Build history of the part. All positions in model axes, mm. A direction names the side the tool comes from. Round coordinates to 2 decimals unless told otherwise and drop trailing zeros. Write each loop counter-clockwise with the first axis right and the second up, starting at its lowest first coordinate (ties: lowest second). Pieces come first, ordered by that corner, then holes.
from build123d import *

# Parameters (mm, degrees)
SKETCH1_W           = 98
SKETCH1_H           = 60
BOSS_EXTRUDE1_DEPTH = 1.5
SKETCH2_W           = 87.5
SKETCH2_H           = 42
BOSS_EXTRUDE2_DEPTH = 9
SKETCH3_W           = 76.5
SKETCH3_H           = 25.4
CUT_EXTRUDE1_DEPTH  = 0.5
SKETCH4_R           = 1.25
CUT_EXTRUDE2_DEPTH  = 116.260574352
SKETCH5_R           = 0.5
CUT_EXTRUDE3_DEPTH  = 10
BOSS_EXTRUDE3_START = 0.1
SKETCH6_R           = 0.75
SKETCH6_R_2         = 0.5
SKETCH6_W           = 1.5
SKETCH6_H           = 1.5
BOSS_EXTRUDE3_DEPTH = 0.1
SKETCH7_R           = 0.75
SKETCH7_R_2         = 0.5
SKETCH7_W           = 1.5
SKETCH7_H           = 1.5
BOSS_EXTRUDE4_DEPTH = 1.7
BOSS_EXTRUDE5_DEPTH = 2.59


with BuildPart() as part:
    # Sketch1 → Boss-Extrude1 (new body)
    with BuildSketch(Plane(origin=(0, 0, 0), x_dir=(1, 0, 0), z_dir=(0, 1, 0))):
        with Locations((49, 30)):
            Rectangle(SKETCH1_W, SKETCH1_H)
    extrude(amount=BOSS_EXTRUDE1_DEPTH)

    # Sketch2 → Boss-Extrude2 (add)
    with BuildSketch(Plane(origin=(0, 1.5, 0), x_dir=(1, 0, 0), z_dir=(0, 1, 0))):
        with Locations((49, 30)):
            Rectangle(SKETCH2_W, SKETCH2_H)
    extrude(amount=BOSS_EXTRUDE2_DEPTH)

    # Sketch3 → Cut-Extrude1 (cut)
    with BuildSketch(Plane(origin=(0, 10.5, 0), x_dir=(1, 0, 0), z_dir=(0, 1, 0))):
        with Locations((49, 30)):
            Rectangle(SKETCH3_W, SKETCH3_H)
    extrude(amount=-CUT_EXTRUDE1_DEPTH, mode=Mode.SUBTRACT)

    # Sketch4 → Cut-Extrude2 (cut, through all)
    with BuildSketch(Plane(origin=(0, 1.5, 0), x_dir=(1, 0, 0), z_dir=(0, 1, 0))):
        with Locations(Location((2.5, 57.5, 0), (0, 0, 270))):
            Circle(SKETCH4_R)
        with Locations(Location((95.5, 57.5, 0), (0, 0, 270))):
            Circle(SKETCH4_R)
        with Locations(Location((95.5, 2.5, 0), (0, 0, 270))):
            Circle(SKETCH4_R)
        with Locations(Location((2.5, 2.5, 0), (0, 0, 270))):
            Circle(SKETCH4_R)
    extrude(amount=-CUT_EXTRUDE2_DEPTH, mode=Mode.SUBTRACT)

    # Sketch5 → Cut-Extrude3 (cut)
    with BuildSketch(Plane(origin=(0, 1.5, 0), x_dir=(1, 0, 0), z_dir=(0, 1, 0))):
        with Locations(Location((10, 57.5, 0), (0, 0, 270))):
            Circle(SKETCH5_R)
        with Locations(Location((12.54, 57.5, 0), (0, 0, 270))):
            Circle(SKETCH5_R)
        with Locations(Location((15.08, 57.5, 0), (0, 0, 270))):
            Circle(SKETCH5_R)
        with Locations(Location((20.16, 57.5, 0), (0, 0, 270))):
            Circle(SKETCH5_R)
        with Locations(Location((22.7, 57.5, 0), (0, 0, 270))):
            Circle(SKETCH5_R)
        with Locations(Location((25.24, 57.5, 0), (0, 0, 270))):
            Circle(SKETCH5_R)
        with Locations(Location((27.78, 57.5, 0), (0, 0, 270))):
            Circle(SKETCH5_R)
        with Locations(Location((30.32, 57.5, 0), (0, 0, 270))):
            Circle(SKETCH5_R)
        with Locations(Location((32.86, 57.5, 0), (0, 0, 270))):
            Circle(SKETCH5_R)
    extrude(amount=-CUT_EXTRUDE3_DEPTH, mode=Mode.SUBTRACT)

    # Sketch6 → Boss-Extrude3 (add)
    # profile 1 of 9: a face of its own
    with BuildSketch(Plane(origin=(0, 1.5, 0), x_dir=(1, 0, 0), z_dir=(0, 1, 0)).offset(BOSS_EXTRUDE3_START)):
        with Locations(Location((12.54, 57.5, 0), (0, 0, 90))):
            Circle(SKETCH6_R)
        with Locations(Location((12.54, 57.5, 0), (0, 0, 270))):
            Circle(SKETCH6_R_2, mode=Mode.SUBTRACT)
    # profile 2 of 9: a face of its own
    with BuildSketch(Plane(origin=(0, 1.5, 0), x_dir=(1, 0, 0), z_dir=(0, 1, 0)).offset(BOSS_EXTRUDE3_START)):
        with Locations(Location((15.08, 57.5, 0), (0, 0, 90))):
            Circle(SKETCH6_R)
        with Locations(Location((15.08, 57.5, 0), (0, 0, 270))):
            Circle(SKETCH6_R_2, mode=Mode.SUBTRACT)
    # profile 3 of 9: a face of its own
    with BuildSketch(Plane(origin=(0, 1.5, 0), x_dir=(1, 0, 0), z_dir=(0, 1, 0)).offset(BOSS_EXTRUDE3_START)):
        with Locations(Location((22.7, 57.5, 0), (0, 0, 90))):
            Circle(SKETCH6_R)
        with Locations(Location((22.7, 57.5, 0), (0, 0, 270))):
            Circle(SKETCH6_R_2, mode=Mode.SUBTRACT)
    # profile 4 of 9: a face of its own
    with BuildSketch(Plane(origin=(0, 1.5, 0), x_dir=(1, 0, 0), z_dir=(0, 1, 0)).offset(BOSS_EXTRUDE3_START)):
        with Locations(Location((25.24, 57.5, 0), (0, 0, 90))):
            Circle(SKETCH6_R)
        with Locations(Location((25.24, 57.5, 0), (0, 0, 270))):
            Circle(SKETCH6_R_2, mode=Mode.SUBTRACT)
    # profile 5 of 9: a face of its own
    with BuildSketch(Plane(origin=(0, 1.5, 0), x_dir=(1, 0, 0), z_dir=(0, 1, 0)).offset(BOSS_EXTRUDE3_START)):
        with Locations(Location((27.78, 57.5, 0), (0, 0, 90))):
            Circle(SKETCH6_R)
        with Locations(Location((27.78, 57.5, 0), (0, 0, 270))):
            Circle(SKETCH6_R_2, mode=Mode.SUBTRACT)
    # profile 6 of 9: a face of its own
    with BuildSketch(Plane(origin=(0, 1.5, 0), x_dir=(1, 0, 0), z_dir=(0, 1, 0)).offset(BOSS_EXTRUDE3_START)):
        with Locations(Location((30.32, 57.5, 0), (0, 0, 90))):
            Circle(SKETCH6_R)
        with Locations(Location((30.32, 57.5, 0), (0, 0, 270))):
            Circle(SKETCH6_R_2, mode=Mode.SUBTRACT)
    # profile 7 of 9: a face of its own
    with BuildSketch(Plane(origin=(0, 1.5, 0), x_dir=(1, 0, 0), z_dir=(0, 1, 0)).offset(BOSS_EXTRUDE3_START)):
        with Locations(Location((32.86, 57.5, 0), (0, 0, 90))):
            Circle(SKETCH6_R)
        with Locations(Location((32.86, 57.5, 0), (0, 0, 270))):
            Circle(SKETCH6_R_2, mode=Mode.SUBTRACT)
    # profile 8 of 9: a face of its own
    with BuildSketch(Plane(origin=(0, 1.5, 0), x_dir=(1, 0, 0), z_dir=(0, 1, 0)).offset(BOSS_EXTRUDE3_START)):
        with Locations((20.16, 57.5)):
            Rectangle(SKETCH6_W, SKETCH6_H)
        with Locations(Location((20.16, 57.5, 0), (0, 0, 270))):
            Circle(SKETCH6_R_2, mode=Mode.SUBTRACT)
    # profile 9 of 9: a face of its own
    with BuildSketch(Plane(origin=(0, 1.5, 0), x_dir=(1, 0, 0), z_dir=(0, 1, 0)).offset(BOSS_EXTRUDE3_START)):
        with Locations((10, 57.5)):
            Rectangle(SKETCH6_W, SKETCH6_H)
        with Locations(Location((10, 57.5, 0), (0, 0, 270))):
            Circle(SKETCH6_R_2, mode=Mode.SUBTRACT)
    extrude(amount=-BOSS_EXTRUDE3_DEPTH)

    # Sketch7 → Boss-Extrude4 (add)
    # profile 1 of 9: a face of its own
    with BuildSketch(Plane(origin=(0, 1.6, 0), x_dir=(1, 0, 0), z_dir=(0, 1, 0))):
        with Locations(Location((12.54, 57.5, 0), (0, 0, 90))):
            Circle(SKETCH7_R)
        with Locations(Location((12.54, 57.5, 0), (0, 0, 270))):
            Circle(SKETCH7_R_2, mode=Mode.SUBTRACT)
    # profile 2 of 9: a face of its own
    with BuildSketch(Plane(origin=(0, 1.6, 0), x_dir=(1, 0, 0), z_dir=(0, 1, 0))):
        with Locations(Location((15.08, 57.5, 0), (0, 0, 90))):
            Circle(SKETCH7_R)
        with Locations(Location((15.08, 57.5, 0), (0, 0, 270))):
            Circle(SKETCH7_R_2, mode=Mode.SUBTRACT)
    # profile 3 of 9: a face of its own
    with BuildSketch(Plane(origin=(0, 1.6, 0), x_dir=(1, 0, 0), z_dir=(0, 1, 0))):
        with Locations(Location((22.7, 57.5, 0), (0, 0, 90))):
            Circle(SKETCH7_R)
        with Locations(Location((22.7, 57.5, 0), (0, 0, 270))):
            Circle(SKETCH7_R_2, mode=Mode.SUBTRACT)
    # profile 4 of 9: a face of its own
    with BuildSketch(Plane(origin=(0, 1.6, 0), x_dir=(1, 0, 0), z_dir=(0, 1, 0))):
        with Locations(Location((25.24, 57.5, 0), (0, 0, 90))):
            Circle(SKETCH7_R)
        with Locations(Location((25.24, 57.5, 0), (0, 0, 270))):
            Circle(SKETCH7_R_2, mode=Mode.SUBTRACT)
    # profile 5 of 9: a face of its own
    with BuildSketch(Plane(origin=(0, 1.6, 0), x_dir=(1, 0, 0), z_dir=(0, 1, 0))):
        with Locations(Location((27.78, 57.5, 0), (0, 0, 90))):
            Circle(SKETCH7_R)
        with Locations(Location((27.78, 57.5, 0), (0, 0, 270))):
            Circle(SKETCH7_R_2, mode=Mode.SUBTRACT)
    # profile 6 of 9: a face of its own
    with BuildSketch(Plane(origin=(0, 1.6, 0), x_dir=(1, 0, 0), z_dir=(0, 1, 0))):
        with Locations(Location((30.32, 57.5, 0), (0, 0, 90))):
            Circle(SKETCH7_R)
        with Locations(Location((30.32, 57.5, 0), (0, 0, 270))):
            Circle(SKETCH7_R_2, mode=Mode.SUBTRACT)
    # profile 7 of 9: a face of its own
    with BuildSketch(Plane(origin=(0, 1.6, 0), x_dir=(1, 0, 0), z_dir=(0, 1, 0))):
        with Locations(Location((32.86, 57.5, 0), (0, 0, 90))):
            Circle(SKETCH7_R)
        with Locations(Location((32.86, 57.5, 0), (0, 0, 270))):
            Circle(SKETCH7_R_2, mode=Mode.SUBTRACT)
    # profile 8 of 9: a face of its own
    with BuildSketch(Plane(origin=(0, 1.6, 0), x_dir=(1, 0, 0), z_dir=(0, 1, 0))):
        with Locations((10, 57.5)):
            Rectangle(SKETCH7_W, SKETCH7_H)
        with Locations(Location((10, 57.5, 0), (0, 0, 270))):
            Circle(SKETCH7_R_2, mode=Mode.SUBTRACT)
    # profile 9 of 9: a face of its own
    with BuildSketch(Plane(origin=(0, 1.6, 0), x_dir=(1, 0, 0), z_dir=(0, 1, 0))):
        with Locations((20.16, 57.5)):
            Rectangle(SKETCH7_W, SKETCH7_H)
        with Locations(Location((20.16, 57.5, 0), (0, 0, 270))):
            Circle(SKETCH7_R_2, mode=Mode.SUBTRACT)
    extrude(amount=-BOSS_EXTRUDE4_DEPTH)

    # Sketch8 → Boss-Extrude5 (add)
    with BuildSketch(Plane.XZ):
        Polygon((5.25, -9), (5.25, -12), (5.75, -12), (5.75, -9.5), (8.25, -9.5), (8.25, -9), align=None)
        Polygon((92.25, -12), (92.75, -12), (92.75, -9), (89.75, -9), (89.75, -9.5), (92.25, -9.5), align=None)
        Polygon((92.75, -51), (92.75, -48), (92.25, -48), (92.25, -50.5), (89.75, -50.5), (89.75, -51), align=None)
        Polygon((5.75, -48), (5.25, -48), (5.25, -51), (8.25, -51), (8.25, -50.5), (5.75, -50.5), align=None)
    extrude(amount=BOSS_EXTRUDE5_DEPTH)


solid = part.part
1) Slice it at B-B (x = 2.5). Write the cut outline in (y, z).
Results:
outline: (0, -60) - (1.5, -60) - (1.5, -58.75) - (0, -58.75) - close; (0, -56.25) - (1.5, -56.25) - (1.5, -3.75) - (0, -3.75) - close; (0, -1.25) - (1.5, -1.25) - (1.5, 0) - (0, 0) - close
2) Wall check: L1, parallel to Z at x = 95.5, y = 1.1; L2, parallel to Y at x = 77.5, z = -50.5; L3, parallel to Z at x = 12, y = 6. Give the ranges that are in metal, low to high.
Results:
L1: z = -60 to -58.75, -56.25 to -3.75, -1.25 to 0
L2: y = 0 to 10.5
L3: z = -51 to -9
3) Which spindle directions (+Z, -Z, +X, -X, +Y, -Y) get a long thin tool onto all of the face, cutting with end or side? Do faces 4 (the flat face through (48, 6, -9)), 5 (the flat face through (7, -1, -51)), 6 (the flat face through (5.25, 6, -30)), 7 (the flat face through (91, -1, -50.5)), 8 (the flat face through (92.75, -1, -50)). Say none if no direction does.
Results:
face 4: +Z, +X, -X, +Y
face 5: -Z, +X, -X, -Y
face 6: +Z, -Z, -X, +Y
face 7: -Y
face 8: +Z, -Z, +X, -Y
4) Pin check, flat tips, straight feed: pin 1 Ø0.8 at (x, z) = (25, -57.5) entering from -Y; pin 2 Ø0.6 at (y, z) = (10, -25.5) entering from -X; pin 3 Ø0.8 at (x, y) = (7, -1) entering from -Z. Stop position of each tip, or through.
Results:
pin 1: stops at y = -0.1
pin 2: stops at x = 5.25
pin 3: stops at z = -51
5) Mould opens along X. For faces 1 (the flat face through (48, 10, -30)), 2 (the flat face through (91, -1, -9)), 3 (the flat face through (92.75, -1, -11)) say: released by +X, released by -X, zero draft, split by the parting line, or undercut.
Results:
face 1: undercut
face 2: zero draft
face 3: released by +X
6) Slice it at A-A (z = -2.5). Write the cut outline in (x, y).
Results:
outline: (0, 0) - (1.25, 0) - (1.25, 1.5) - (0, 1.5) - close; (3.75, 0) - (94.25, 0) - (94.25, 1.5) - (3.75, 1.5) - close; (96.75, 0) - (98, 0) - (98, 1.5) - (96.75, 1.5) - close
7) Slice it at D-D (y = 3). Write the cut outline in (x, z).
Results:
outline: (5.25, -51) - (92.75, -51) - (92.75, -9) - (5.25, -9) - close
8) Slice it at C-C (z = -38.5). Write the cut outline in (x, y), plus the area to 3 significant figures.
Results:
outline: (0, 0) - (98, 0) - (98, 1.5) - (92.75, 1.5) - (92.75, 10.5) - (87.25, 10.5) - (87.25, 10) - (10.75, 10) - (10.75, 10.5) - (5.25, 10.5) - (5.25, 1.5) - (0, 1.5) - close
area: 896 mm2
